```python
from build123d import *

# Parameters (mm, degrees)
CHAMFER_1_SIZE      = 1
CUT_EXTRUDE_START   = -17.5
CUT_EXTRUDE_1_DEPTH = 5


with BuildPart() as part:
    # Эскиз1 → Повернуть1 (revolve)
    with BuildSketch(Plane.XY, mode=Mode.PRIVATE) as revolve_1_sk:
        Polygon((0, 0), (0, 17.5), (56, 17.5), (56, 20), (85, 20), (85, 25), (145.5, 25), (145.5, 32.5), (153, 32.5), (153, 28.5), (203, 28.5), (203, 0), align=None)
    revolve(revolve_1_sk.sketch.rotate(Axis((0, 0, 0), (1, 0, 0)), 90), axis=Axis((0, 0, 0), (1, 0, 0)))

    # Фаска1
    chamfer_1_edges = [part.edges().sort_by_distance(p)[0] for p in [
        (153, 0, -32.5),
        (145.5, 0, -32.5),
        (85, 0, -25),
        (56, 0, -20),
        (0, 0, -17.5),
        (203, 0, -28.5),
    ]]
    chamfer(chamfer_1_edges, length=CHAMFER_1_SIZE)

    # Эскиз2 → Вырез-Вытянуть1 (cut)
    with BuildSketch(Plane.XY.offset(CUT_EXTRUDE_START)):
        with BuildLine():
            Line((7, 5), (47, 5))
            ThreePointArc((47, 5), (52, 0), (47, -5))
            Line((47, -5), (7, -5))
            ThreePointArc((7, -5), (2, 0), (7, 5))
        make_face()
    extrude(amount=CUT_EXTRUDE_1_DEPTH, mode=Mode.SUBTRACT)


solid = part.part
```
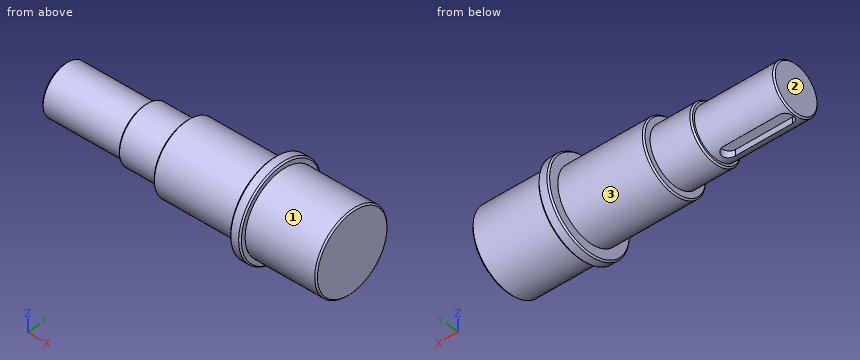
The model under review builds one solid part; all positions refer to its coordinate system, in mm. Face numbers are marked on the shaded views. A direction names the side the tool comes from. Round coordinates to 2 decimals unless told otherwise and drop trailing zeros. Loops run counter-clockwise (first coordinate to the right, second up) from the corner with the lowest first, then second, coordinate; pieces in that order, holes last. Notation, with made-up numbers: (35.5, 15) - (76.5, 15) arc R14 ccw to (76.5, 33) - close; hole circle Ø7 at (83.25, 71). An arc over 180 degrees is marked (long way). Use a Markdown table: item, result. Add a question column.
Q1. Add section C-C (x = 31). State the section outline as (y, z) points.
Q2. Add section B-B (x = 155). State the section outline as (y, z) points.
Q3. Machinability: for the marked faces 1, 2 and 3, which of the approach directions +Z, -Z, +X, -X, +Y, -Y give a long, thin tool a straight path to every point of the face, cutting with its end or side? Answer none if there is none.
Q4. Insertion check: pin 1 Ø3 at (y, z) = (-19, 16) entering from -X; pin 2 Ø3 at (x, y) = (35.5, -1.5) entering from -Z; pin 3 Ø1.5 at (x, z) = (131.5, -8.5) entering from +Y. Each pin has a flat end and moves straight along its axis. Give the tip position at first contact, or say it passes through.
Q5. For probe 1 along X at (y, z) = (-10.5, -27); probe 2 along X at (y, z) = (4, 18.5); probe 3 along Z at (x, y) = (37.5, -10.5), list the stretches that pass through material, from the lowest coordinate up.
Worked answers:
| question | item | result |
|---|---|---|
| 1 | outline | (-5, -16.77) - (-5, -12.5) - (5, -12.5) - (5, -16.77) arc R17.5 ccw (long way) to start |
| 2 | outline | circle Ø57 at (0, 0) |
| 3 | face 1 | +X |
| 3 | face 2 | +Z, -Z, -X, +Y, -Y |
| 3 | face 3 | -X |
| 4 | pin 1 | x = 85 |
| 4 | pin 2 | z = -12.5 |
| 4 | pin 3 | y = 23.77 |
| 5 | probe 1 | 145.5 to 153 |
| 5 | probe 2 | 56 to 203 |
| 5 | probe 3 | -14 to 14 |
